CAD build for the part. Positions are in the model's coordinates, mm. A direction names the side the tool comes from. Round coordinates to 2 decimals unless told otherwise and drop trailing zeros. Loops run counter-clockwise (first coordinate to the right, second up) from the corner with the lowest first, then second, coordinate; pieces in that order, holes last. Notation, with made-up numbers: M 83,-19 L 119,-19 A10 cw 119,-8 Z; hole C 4.25,56.5 d5. An arc over 180 degrees is marked long. Use a Markdown table: item, result. Add a question column.
(1) Which spindle directions (+Z, -Z, +X, -X, +Y, -Y) get a long thin tool onto all of the face, cutting with end or side? Do faces 4 (the face through (-65, 14, -21)), 5 (the face through (41, 8, -15)), 6 (the face through (-31.1, 8.86, -33.27)). Say none if no direction does.
(2) Band-saw the part on D-D, the plane x = 49. Write the cut outline in (y, z), and give its area (3 significant figures).
(3) Band-saw the part on B-B, the plane z = -7. Write the cut outline in (x, y), and give its area (3 significant figures).
(4) Wall check: L1, parallel to Z at x = 0, y = 27; L2, parallel to X at y = 0, z = -13; L3, parallel to Y at x = 0, z = -18.5. Give the ranges that are in metal, low to high.
(5) Flat gauge pins, fed straight in: P1, Ø12, axis at x = 17.5, z = -17.5, coming from the -Y side; P2, Ø19, axis at x = 53.5, z = -19.5, coming from the +Y side; P3, Ø2, axis at y = -15, z = -16.5, coming from the -X side. Where does each tip first touch, or does it go through?
(6) Two-plate mould, pull along Y, no slides. Class faces 1 (the face through (-2.75, -12.39, -2.81)), 2 (the face through (-33, 18, -35)), 3 (the face through (-43, -10, -26)): released by +Y, released by -Y, zero draft, split by the parting line, or undercut.
(7) Band-saw the part on A-A, the plane y = 0. Write the cut outline in (x, z), and give its area (3 significant figures).
(8) Band-saw the part on C-C, the plane x = 0. Write the cut outline in (y, z), and give its area (3 significant figures).
from build123d import *

# Parameters (mm, degrees)
SKETCH1_R               = 12.5
BOSS_EXTRUDE1_DEPTH     = 50
SKETCH2_W               = 35
SKETCH2_H               = 30
BOSS_EXTRUDE2_DEPTH     = 30
CUT_EXTRUDE1_DEPTH      = 92.021975369
CUT_EXTRUDE1_DEPTH_BACK = 92.021975369
FILLET2_R               = 3
CHAMFER1_SIZE           = 3


# Read off the part's stored shape, not the designer's step: Ø5.5 (5.5) Diameter Hole1
with BuildPart() as part:
    # Sketch1 → Boss-Extrude1 (new body)
    with BuildSketch(Plane.XY):
        with BuildLine():
            Line((23, 8), (67, 8))
            Line((67, 8), (67, -10))
            Line((67, -10), (20.155644371, -10))
            ThreePointArc((20.155644371, -10), (0, -22.5), (-20.155644371, -10))
            Line((-20.155644371, -10), (-67, -10))
            Line((-67, -10), (-67, 8))
            Line((-67, 8), (-23, 8))
            Line((-23, 8), (-23, 36))
            Line((-23, 36), (23, 36))
            Line((23, 36), (23, 8))
        make_face()
        Circle(SKETCH1_R, mode=Mode.SUBTRACT)
    extrude(amount=-BOSS_EXTRUDE1_DEPTH)

    # Sketch2 → Boss-Extrude2 (add)
    with BuildSketch(Plane.XZ.offset(10)):
        with Locations((49.5, -35)):
            Rectangle(SKETCH2_W, SKETCH2_H)
        with Locations((-49.5, -35)):
            Rectangle(SKETCH2_W, SKETCH2_H)
    extrude(amount=-BOSS_EXTRUDE2_DEPTH)

    # Sketch3 → Cut-Extrude1 (cut, two sides: drawn at the far end of the back side and taken through both)
    with BuildSketch(Plane(origin=(0, 0, 0), x_dir=(1, 0, 0), z_dir=(0, 1, 0)).offset(-CUT_EXTRUDE1_DEPTH_BACK)):
        with BuildLine():
            Line((-32, 50), (-32, 55))
            Line((-32, 55), (32, 55))
            Line((32, 55), (32, 50))
            ThreePointArc((32, 50), (0, 35.202941017), (-32, 50))
        make_face()
    extrude(amount=CUT_EXTRUDE1_DEPTH + CUT_EXTRUDE1_DEPTH_BACK, mode=Mode.SUBTRACT)

    # Ø5.5 (5.5) Diameter Hole1 outline → Ø5.5 (5.5) Diameter Hole1 (revolve, cut)
    with BuildSketch(Plane.XY.offset(-14.276580189)):
        Polygon((0, 12.193702386), (2.75, 12.193702386), (2.75, 33.55), (5.2, 36), (0, 36), align=None)
    revolve(axis=Axis((0, 0, -14.276580189), (0, 1, 0)), mode=Mode.SUBTRACT)

    # Fillet2
    fillet2_edges = [part.edges().sort_by_distance(p)[0] for p in [
        (49.5, 8, -20),
        (-49.5, 8, -20),
        (-32, 8, -35),
        (32, 8, -35),
        (23, 8, -21.030187118),
        (-23, 8, -21.030187118),
        (20.155644371, -10, -20.177640831),
        (-20.155644371, -10, -20.177640831),
    ]]
    fillet(fillet2_edges, radius=FILLET2_R)

    # Chamfer1
    chamfer1_edges = [part.edges().sort_by_distance(p)[0] for p in [
        (-23, 23.5, 0),
        (0, 36, 0),
        (46.5, 8, 0),
        (67, -1, 0),
        (67, 8, -8.5),
        (-67, 8, -8.5),
        (-46.5, 8, 0),
        (23, 23.5, 0),
        (0, -22.5, 0),
        (-44.468705484, -10, 0),
        (44.468705484, -10, 0),
        (67, 8.878679656, -19.121320344),
        (-67, 8.878679656, -19.121320344),
        (-67, -1, 0),
        (23.878679656, 8.878679656, 0),
        (-23.878679656, 8.878679656, 0),
        (20.452189654, -10.393447172, 0),
        (-20.452189654, -10.393447172, 0),
        (67, -10, -25),
        (-67, -10, -25),
        (-12.5, 0, 0),
        (67, 15.5, -20),
        (32, 20, -35),
        (49.5, 20, -20),
        (-32, 20, -35),
        (-67, 15.5, -20),
        (-49.5, 20, -20),
    ]]
    chamfer(chamfer1_edges, length=CHAMFER1_SIZE)


solid = part.part
Return value:
| question | item | result |
|---|---|---|
| 1 | face 4 | +Z, -X, +Y |
| 1 | face 5 | +Z, +Y |
| 1 | face 6 | +Z, -Z, +Y |
| 2 | outline | M -10,-50 L 20,-50 L 20,-23 L 17,-20 L 11,-20 A3 cw 8,-17 L 8,-3 L 5,0 L -7,0 L -10,-3 Z |
| 2 | area | 1,250 mm^2 |
| 3 | outline | M -67,-7 L -64,-10 L -21.94,-10 A3 cw -19.36,-11.47 A22.5 ccw 19.36,-11.47 A3 cw 21.94,-10 L 64,-10 L 67,-7 L 67,5 L 64,8 L 26,8 A3 cw 23,11 L 23,36 L -23,36 L -23,11 A3 cw -26,8 L -64,8 L -67,5 Z; hole C 0,0 d25 |
| 3 | area | 3,560 mm^2 |
| 4 | L1 | -35.2 to -17.03, -11.53 to 0 |
| 4 | L2 | -67 to -12.5, 12.5 to 67 |
| 4 | L3 | -22.5 to -12.5, 12.5 to 35.02 |
| 5 | P1 | y = -19.34 |
| 5 | P2 | y = 20 |
| 5 | P3 | x = -17.61 |
| 6 | face 1 | undercut |
| 6 | face 2 | released by +Y |
| 6 | face 3 | released by -Y |
| 7 | outline | M -67,-50 L -32,-50 A42 cw -12.5,-37.11 L -12.5,-3 L -15.5,0 L -64,0 L -67,-3 Z; M 12.5,-37.11 A42 cw 32,-50 L 67,-50 L 67,-3 L 64,0 L 15.5,0 L 12.5,-3 Z |
| 7 | area | 5,130 mm^2 |
| 8 | outline | M -22.5,-35.2 L -12.5,-35.2 L -12.5,-3 L -15.5,0 L -19.5,0 L -22.5,-3 Z; M 12.5,-35.2 L 36,-35.2 L 36,-19.48 L 33.55,-17.03 L 12.5,-17.03 Z; M 12.5,-11.53 L 33.55,-11.53 L 36,-9.08 L 36,-3 L 33,0 L 15.5,0 L 12.5,-3 Z |
| 8 | area | 1,030 mm^2 |
